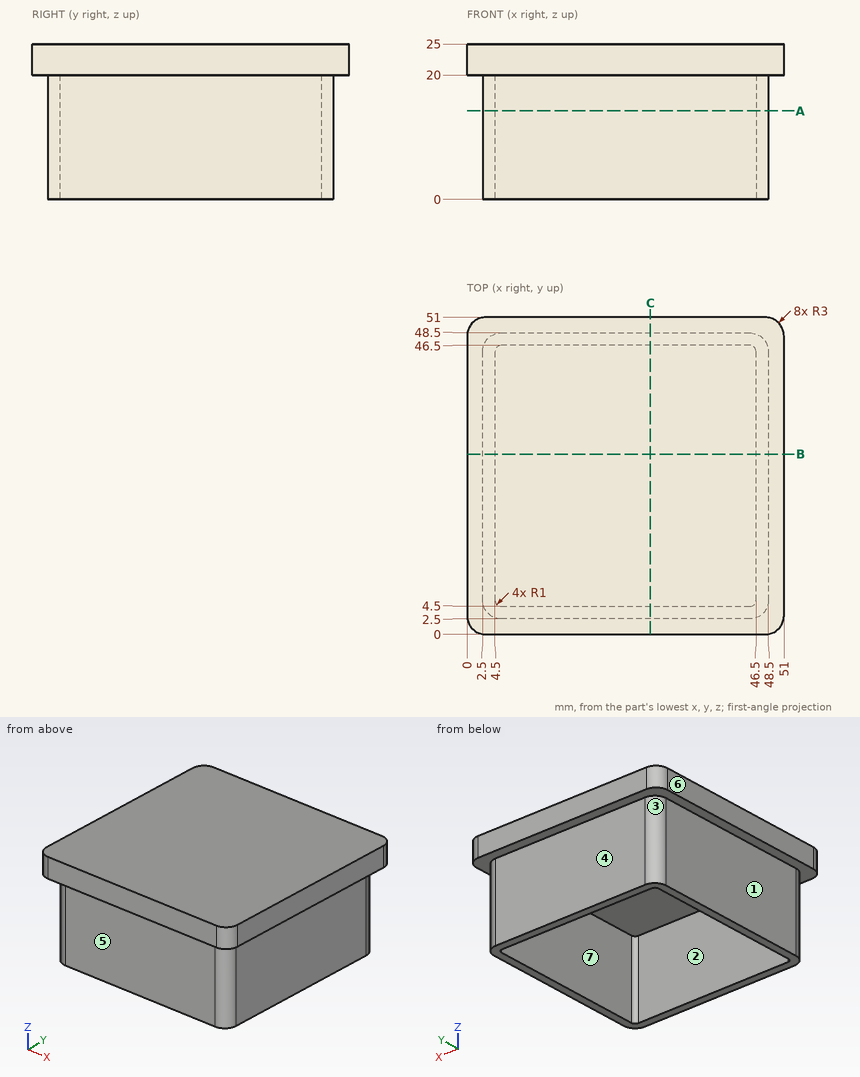
Design review of the part shown in the three views and the two pictorial views. Dimensions are in mm from the part's minimum x, y and z. A direction names the side the tool comes from. Round coordinates to 2 decimals unless told otherwise and drop trailing zeros. Order: outer loops, then holes, each group sorted by start corner. A loop starts at its lowest first (then second) coordinate and runs counter-clockwise, first axis right, second up. Notation, with made-up numbers: (22, 63.5) -> (58, 63.5) arc R22 ccw to (58, 101.5) -> close; hole circle Ø10 at (-7, 57). An arc over 180 degrees is marked (long way). Write item = value, one per line. Start each with the question number.
1) Tool access review of the marked faces 1, 2, 3 and 4: name each direction out of +Z, -Z, +X, -X, +Y, -Y from which nothing blocks a thin tool from reaching the whole face with its end or side.
2) Take a section at A-A on z = 14.25. State the section outline as (x, y) points.
3) To check wall thickness, follow line 1 (Y direction, x = 8, z = 19); line 2 (Z direction, x = 35, y = 21). State the ranges of each line that lie inside material, in increasing order. Write a range as from..to.
4) Take a section at B-B on y = 29. State the section outline as (x, z) points, plus the area to 3 significant figures.
5) Insertion check: pin 1 (5 mm diameter, centred on x = 10.5, y = 11, fed in from -Z); pin 2 (6 mm diameter, centred on y = 31.5, z = 12.5, fed in from -X); pin 3 (6 mm diameter, centred on x = 32.5, z = 8, fed in from +Y); pin 4 (12 mm diameter, centred on x = 7, z = 19.5, fed in from -Y). Each pin has a flat end and moves straight along its axis. Give the tip position at first contact, or say it passes through.
6) The part is to be moulded in two halves that separate along Y. For the marked faces 5, 6 and 7, say which applies: +Y half, -Y half, draft (parallel to the pull), parting line (faces both ways), or undercut.
Verdict:
q1.face_1 = -Z, -X, +Y, -Y
q1.face_2 = -Z
q1.face_3 = -Z, -X, +Y
q1.face_4 = -Z, +X, -X, +Y
q2.outline = (2.5, 5.5) arc R3 ccw to (5.5, 2.5) -> (45.5, 2.5) arc R3 ccw to (48.5, 5.5) -> (48.5, 45.5) arc R3 ccw to (45.5, 48.5) -> (5.5, 48.5) arc R3 ccw to (2.5, 45.5) -> close; hole (4.5, 5.5) arc R1 ccw to (5.5, 4.5) -> (45.5, 4.5) arc R1 ccw to (46.5, 5.5) -> (46.5, 45.5) arc R1 ccw to (45.5, 46.5) -> (5.5, 46.5) arc R1 ccw to (4.5, 45.5) -> close
q3.line_1 = 2.5..4.5, 46.5..48.5
q3.line_2 = 20..25
q4.outline = (0, 20) -> (2.5, 20) -> (2.5, 0) -> (4.5, 0) -> (4.5, 20) -> (46.5, 20) -> (46.5, 0) -> (48.5, 0) -> (48.5, 20) -> (51, 20) -> (51, 25) -> (0, 25) -> close
q4.area = 335 mm2
q5.pin_1 = 20
q5.pin_2 = 2.5
q5.pin_3 = 48.5
q5.pin_4 = 0
q6.face_5 = -Y half
q6.face_6 = draft
q6.face_7 = undercut
